The model under review builds one solid part; all positions refer to its coordinate system, in mm. Face numbers are marked on the shaded views. A direction names the side the tool comes from. Round coordinates to 2 decimals unless told otherwise and drop trailing zeros. Order: outer loops, then holes, each group sorted by start corner. A loop starts at its lowest first (then second) coordinate and runs counter-clockwise, first axis right, second up. Notation, with made-up numbers: M 64.5,-14.5 L 116.5,-14.5 A21 ccw 116.5,-10.5 Z; hole C 24,10 d1. An arc over 180 degrees is marked long. Answer as a JSON object with one key per item and string values. Group by question number.
1. Machinability: for the marked faces 4, 5 and 6, which of the approach directions +Z, -Z, +X, -X, +Y, -Y give a long, thin tool a straight path to every point of the face, cutting with its end or side? Answer none if there is none.
2. Add section B-B on y = 11. State the section outline as (x, z) points, and give its area (3 significant figures).
3. To check wall thickness, follow probe 1 along X at (y, z) = (21, 0); probe 2 along Z at (x, y) = (0, 3); probe 3 along Z at (x, y) = (0, 9.25). State the ranges of each line that lie inside material, in increasing order. Write a range as [from, to].
4. Add section C-C on y = 3.75. State the section outline as (x, z) points.
5. Add section A-A on y = 18. State the section outline as (x, z) points.
6. Clearance check with flat-ended pins moving along their axes: P1, Ø8, axis at x = 0, z = 0, coming from the -Y side; P2, Ø3.5, axis at x = 1.5, z = 0, coming from the +Y side; P3, Ø3, axis at x = -3, y = 19.5, coming from the -Z side; P4, Ø1, axis at x = 2, y = 12, coming from the +Z side. State where each tip first meets the part, or that it passes through.
7. Mouldability with a two-part tool opening along Z and no side actions: class the marked faces 1, 2 and 3 as released by +Z, released by -Z, zero draft, split by the parting line, or undercut.
Autodesk Inventor part; units mm, degrees
ref_plane "YZ Plane" through (0, 0, 0) normal (1, 0, 0) x (0, 1, 0)
ref_plane "XZ Plane" through (0, 0, 0) normal (0, 1, 0) x (-1, 0, 0)
ref_plane "XY Plane" through (0, 0, 0) normal (0, 0, 1) x (1, 0, 0)
sketch "Sketch1" plane through (0, 0, 0) normal (0, 1, 0) x (-1, 0, 0)
  circle A0 centre (0, 0) radius 5
  circle A1 centre (0, 0) radius 3.5
  dimension "d0" = 10
  dimension "d1" = 7
extrude "Extrusion1" add sketch "Sketch1" along normal blind 8
sketch "Sketch2" plane through (0, 8, 0) normal (0, 1, 0) x (1, 0, 0)
  circle A0 centre (0, 0) radius 7
  circle A1 centre (0, 0) radius 5
  circle A2 centre (0, 0) radius 3.5
  dimension "d4" = 14
extrude "Extrusion2" add sketch "Sketch2" along normal blind 4 contours A0 | A1
sketch "Sketch3" plane through (0, 12, 0) normal (0, 1, 0) x (1, 0, 0)
  line L0 (-7.483, 4.3203) -> (0, 8.6406)
  line L1 (0, 8.6406) -> (7.483, 4.3203)
  line L2 (7.483, 4.3203) -> (7.483, -4.3203)
  line L3 (7.483, -4.3203) -> (0, -8.6406)
  line L4 (0, -8.6406) -> (-7.483, -4.3203)
  line L5 (-7.483, -4.3203) -> (-7.483, 4.3203)
  circle A0 centre (0, 0) radius 5
extrude "Extrusion3" add sketch "Sketch3" along normal blind 10
sketch "Sketch4" plane through (0, 22, 0) normal (0, 1, 0) x (1, 0, 0)
  circle A0 centre (0, 0) radius 3.5
  circle A1 centre (0, 0) radius 7
  circle A2 centre (0, 0) radius 5
  circle A3 centre (0, 0) radius 5
  dimension "d9" = 14
extrude "Extrusion4" add sketch "Sketch4" along normal blind 2 contours A1
sketch "Sketch5" plane through (0, 24, 0) normal (0, 1, 0) x (1, 0, 0)
  circle A0 centre (0, 0) radius 6.25
  circle A1 centre (0, 0) radius 5
  dimension "d12" = 12.5
extrude "Extrusion5" add sketch "Sketch5" along normal blind 1.5
fillet "Fillet1" radius 2 1 edges at (-6.25, 24, 0)
thread "Thread1"
sketch "Sketch6" plane through (0, 25.5, 0) normal (0, 1, 0) x (1, 0, 0)
  circle A0 centre (0, 0) radius 5.5
  dimension "d18" = 11
extrude "Extrusion6" cut sketch "Sketch6" against normal blind 13.5
sketch "Sketch7" plane through (0, 25.5, 0) normal (0, 1, 0) x (1, 0, 0)
  circle A0 centre (0, 0) radius 5.5
properties part number "entrada_manguera_alicat_presion"
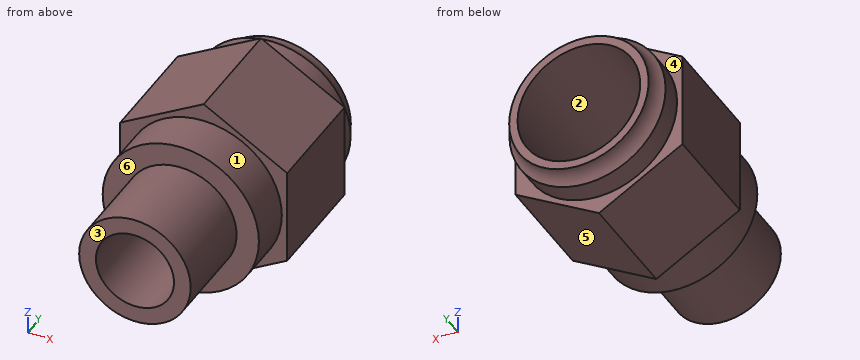
Recorded:
{
 "1": {"face 4": "+Y", "face 5": "-Z, +X, +Y, -Y", "face 6": "-Y"},
 "2": {"outline": "C 0,0 d14; hole C 0,0 d7", "area": "115 mm²"},
 "3": {"probe 1": "x = [-7.48, -5.5], [5.5, 7.48]", "probe 2": "z = [-5, -3.5], [3.5, 5]", "probe 3": "z = [-7, -3.5], [3.5, 7]"},
 "4": {"outline": "C 0,0 d10; hole C 0,0 d7"},
 "5": {"outline": "M -7.48,-4.32 L 0,-8.64 L 7.48,-4.32 L 7.48,4.32 L 0,8.64 L -7.48,4.32 Z; hole C 0,0 d11"},
 "6": {"P1": "stops at y = 0", "P2": "passes through", "P3": "stops at z = -7.77", "P4": "stops at z = 7.77"},
 "7": {"face 1": "split by the parting line", "face 2": "undercut", "face 3": "zero draft"}
}
